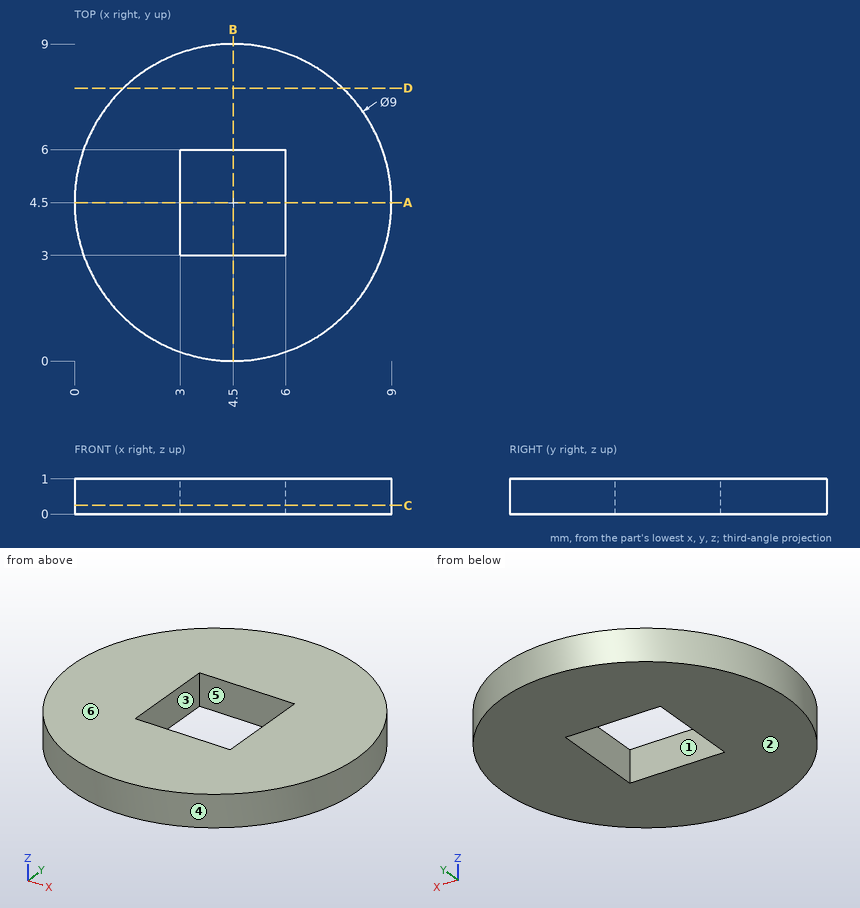
Check sheet for the drawn part. Datum: minimum x, y, z corner. Units: mm. A direction names the side the tool comes from. Give positions to 0.01 mm unless a question says otherwise; leave off trailing zeros. Loops run counter-clockwise (first coordinate to the right, second up) from the corner with the lowest first, then second, coordinate; pieces in that order, holes last.
1) Sectioned sample at C-C, the plane z = 0.25. Enter the section's corners in (x, y).
2) Depth check by flat-ended pin: pin 1 Ø0.5 at (x, z) = (5, 0.5) entering from +Y. Enter the tip coordinate at first touch or a pass-through.
3) Sectioned sample at D-D, the plane y = 7.75. Enter the section's corners in (x, z), then the cut area to 3 significant figures.
4) Set-up check for the marked faces 1 and 2: record each of +Z, -Z, +X, -X, +Y, -Y from which the full face is reachable in a straight line by a thin tool's end or side.
5) Sectioned sample at A-A, the plane y = 4.5. Enter the section's corners in (x, z), then the cut area to 3 significant figures.
6) Draft check along X on the marked faces 3, 4, 5 and 6. Enter one of: pulls with the +X half, pulls with the -X half, needs draft (parallel to the pull), parting line crosses it, or undercut.
7) Thickness scan on line 1 along Y through (x, z) = (4.5, 0.2); line 2 along X through (y, z) = (5, 0.4); line 3 along X through (y, z) = (3.5, 0.3). Record the ranges inside material, lowest first.
Answers:
1. outline: circle Ø9 at (4.5, 4.5); hole (3, 3) - (6, 3) - (6, 6) - (3, 6) - close
2. pin 1: stops at y = 8.99
3. outline: (1.39, 0) - (7.61, 0) - (7.61, 1) - (1.39, 1) - close
3. area: 6.22 mm2
4. face 1: +Z, -Z
4. face 2: -Z, +X, -X, +Y, -Y
5. outline: (0, 0) - (3, 0) - (3, 1) - (0, 1) - close; (6, 0) - (9, 0) - (9, 1) - (6, 1) - close
5. area: 6.00 mm2
6. face 3: undercut
6. face 4: parting line crosses it
6. face 5: undercut
6. face 6: needs draft
7. line 1: y = 0 to 3, 6 to 9
7. line 2: x = 0.03 to 3, 6 to 8.97
7. line 3: x = 0.11 to 3, 6 to 8.89
